The listing builds one solid part. Answer for the finished solid, in the listing's coordinates (mm). Face numbers are marked on the shaded views. A direction names the side the tool comes from. Coordinates: 2 decimals unless noted, no trailing zeros. Loops run counter-clockwise (first coordinate to the right, second up) from the corner with the lowest first, then second, coordinate; pieces in that order, holes last. Notation, with made-up numbers: M -28.5,47.5 L -3.5,47.5 A16 cw -3.5,65.5 Z; hole C 19,30 d6. An arc over 180 degrees is marked long. Answer in a Markdown table with one row per item. Add a question column.
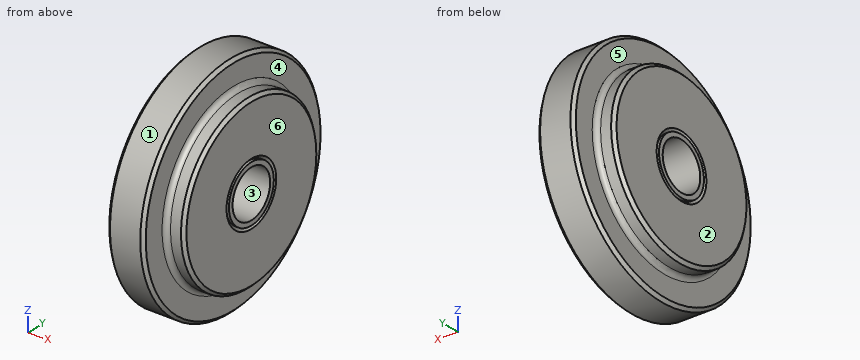
Autodesk Inventor part; units mm, degrees
ref_plane "to_bolt_XY" through (6.096, 0, 0) normal (1, 0, 0) x (0, 0, -1)
ref_plane "to_bolt_YZ" through (6.096, 0, 0) normal (0, 0, -1) x (0, 1, 0)
ref_plane "to_bolt_ZX" through (6.096, 0, 0) normal (0, 1, 0) x (1, 0, 0)
sketch "Sketch_1" plane through (0, 0, 0) normal (0, 0, 1) x (1, 0, 0)
  line L0 (6.096, 0) -> (-6.096, 0)
  line L1 (-6.096, 5.2705) -> (-5.588, 4.7625)
  line L2 (-5.588, 4.7625) -> (5.588, 4.7625)
  line L3 (5.588, 4.7625) -> (6.096, 5.2705)
  line L4 (6.096, 5.2705) -> (6.096, 13.7795)
  line L5 (6.096, 13.7795) -> (5.588, 14.2875)
  line L6 (5.588, 14.2875) -> (3.8354, 14.2875)
  arc A0 (3.048, 15.0749) -> (3.8354, 14.2875) centre (3.8354, 15.0749) ccw
  line L7 (3.048, 15.0749) -> (3.048, 18.542)
  line L8 (3.048, 18.542) -> (2.54, 19.05)
  line L9 (2.54, 19.05) -> (-2.54, 19.05)
  line L10 (-2.54, 19.05) -> (-3.048, 18.542)
  line L11 (-3.048, 18.542) -> (-3.048, 15.0749)
  arc A1 (-3.8354, 14.2875) -> (-3.048, 15.0749) centre (-3.8354, 15.0749) ccw
  line L12 (-3.8354, 14.2875) -> (-5.588, 14.2875)
  line L13 (-5.588, 14.2875) -> (-6.096, 13.7795)
  line L14 (-6.096, 13.7795) -> (-6.096, 5.2705)
revolve "Revolution1" add sketch "Sketch_1" angle 360 about axis through (6.096, 0, 0) along (1, 0, 0)
sketch "Sketch_2" plane through (0, 0, 0) normal (0, 0, 1) x (1, 0, 0)
  line L0 (6.096, 0) -> (-6.096, 0)
  line L1 (-6.096, 4.7625) -> (-6.096, 3.9878)
  line L2 (-6.096, 3.9878) -> (6.096, 3.9878)
  line L3 (6.096, 3.9878) -> (6.096, 4.7625)
  line L4 (6.096, 4.7625) -> (-6.096, 4.7625)
revolve "Revolution2" add sketch "Sketch_2" angle 360 about axis through (6.096, 0, 0) along (1, 0, 0)
ref_plane "to_bolt_XY" through (6.096, 0, 0) normal (1, 0, 0) x (0, 0, -1)
ref_plane "to_bolt_YZ" through (6.096, 0, 0) normal (0, 0, -1) x (0, 1, 0)
ref_plane "to_bolt_ZX" through (6.096, 0, 0) normal (0, 1, 0) x (1, 0, 0)
ref_plane "wheel_XY" through (0, 0, 0) normal (1, 0, 0) x (0, 0, -1)
ref_plane "wheel_YZ" through (0, 0, 0) normal (0, 0, -1) x (0, 1, 0)
ref_plane "wheel_ZX" through (0, 0, 0) normal (0, 1, 0) x (1, 0, 0)
properties part number "2281_w"
(1) A cutting plane is placed at A-A (x = 0.75). Give the vertices of the cut face in (y, z), plus the area to 3 significant figures.
(2) For the marked faces 4, 5 and 6, determine the directions among +Z, -Z, +X, -X, +Y, -Y from which every point of the face is accessible in a straight line to the end or side of a thin tool.
(3) Straight lines are drawn through the part: line 1 (Z direction, x = 1.25, y = 0); line 2 (Z direction, x = 2.5, y = -2.5); line 3 (Y direction, x = -0.75, z = -1). For each, find the intervals that lie inside material, in ascending order.
(4) The mould has two halves that part along Y. Classify the marked faces 1, 2 and 3: released by +Y, released by -Y, zero draft, split by the parting line, or undercut.
(5) Each of these flat-tipped pins is pushed along its axis until it touches: pin 1 (3 mm diameter, centred on y = -15, z = 10.5, fed in from +X); pin 2 (2 mm diameter, centred on x = -1.5, z = -1, fed in from +Y); pin 3 (5 mm diameter, centred on x = 2, y = 10, fed in from -Z); pin 4 (5 mm diameter, centred on x = -4, z = -7, fed in from +Y). Where does it stop, or does it pass through?
Solved:
| question | item | result |
|---|---|---|
| 1 | outline | C 0,0 d38.1; hole C 0,0 d7.98 |
| 1 | area | 1,090 mm² |
| 2 | face 4 | +X |
| 2 | face 5 | -X |
| 2 | face 6 | +Z, -Z, +X, +Y, -Y |
| 3 | line 1 | z = -19.05 to -3.99, 3.99 to 19.05 |
| 3 | line 2 | z = -18.89 to -3.11, 3.11 to 18.89 |
| 3 | line 3 | y = -19.02 to -3.86, 3.86 to 19.02 |
| 4 | face 1 | split by the parting line |
| 4 | face 2 | zero draft |
| 4 | face 3 | undercut |
| 5 | pin 1 | stops at x = 3.05 |
| 5 | pin 2 | stops at y = 19.05 |
| 5 | pin 3 | stops at z = -17.51 |
| 5 | pin 4 | stops at y = 18.39 |
